Geometry check sheet. Reference: the model listing, model coordinates, mm. Face numbers are marked on the shaded views. Coordinates: 2 decimals unless noted, no trailing zeros. Write each loop counter-clockwise with the first axis right and the second up, starting at its lowest first coordinate (ties: lowest second). Pieces come first, ordered by that corner, then holes. Notation, with made-up numbers: (74.5, 40.5) -> (110.5, 40.5) arc R12 ccw to (110.5, 58.5) -> close; hole circle Ø5 at (12, -12). An arc over 180 degrees is marked (long way). Answer in a Markdown table with one row per item. Add a question column.
Q1. Thickness scan on line 1 (Y direction, x = 0, z = 1); line 2 (X direction, y = 1, z = 8.5); line 3 (Y direction, x = 0, z = 18). Record the ranges inside material, lowest first.
Q2. Gauge pin test, flat ends, axial feed: P1, Ø1, axis at x = 16, z = 15.5, coming from the +Y side; P2, Ø18, axis at x = 0, y = 158, coming from the +Z side (1 decimal); P3, Ø1, axis at x = 80, y = 16, coming from the -Z side; P4, Ø2, axis at x = 62.5, z = -7.5, coming from the -Y side. Record the tip position at first contact, or that the pin passes through.
Q3. Section check A-A, the plane x = 0. Record the boundary of the cut face in (y, z), and give its area (3 significant figures).
Q4. Section check B-B, the plane z = 15. Record the boundary of the cut face in (x, y), and give its area (3 significant figures).
Q5. Release check for a two-part mould opening along Y. For the marked faces 1, 2, 3 and 4 record: pulls with the +Y half, pulls with the -Y half, needs draft (parallel to the pull), parting line crosses it, or undercut.
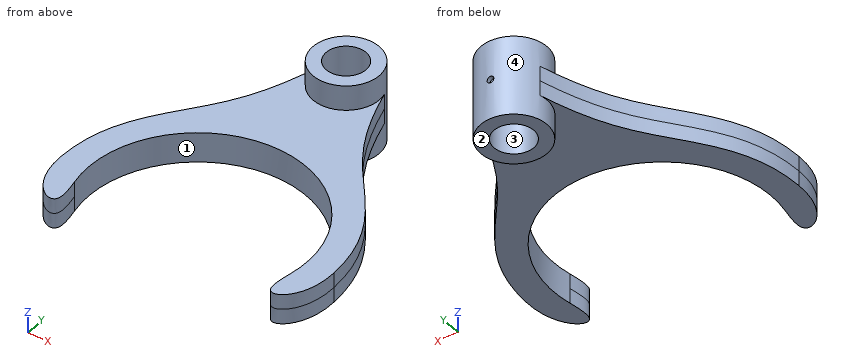
```python
from build123d import *

# Parameters (mm, degrees)
BOSS_EXTRUDE1_DEPTH = 11.25
SKETCH1_3_R         = 25
SKETCH1_3_R_2       = 15
BOSS_EXTRUDE2_DEPTH = 30
SKETCH3_R           = 2.5
CUT_EXTRUDE1_DEPTH  = 4


with BuildPart() as part:
    # Sketch1 → Boss-Extrude1 (new body, symmetric)
    with BuildSketch(Plane.XY):
        with BuildLine():
            ThreePointArc((-80.369346148, -16.271699348), (0, 82), (80.369346148, -16.271699348))
            add(Edge.make_bspline(
                [(101.737711244, 0), (102.498129601, -29.89988011), (76.506237686, -48.322432058), (78.198626966, -26.993338043), (80.369346148, -16.271699348)],
                knots=[0, 0, 0, 0, 0.676560131, 1, 1, 1, 1], degree=3))
            add(Edge.make_bspline(
                [(101.737711244, 0), (100.620263928, 43.938366918), (64.346417004, 80.312533322), (34.633446861, 126.224897928), (24.110391918, 164.609765621)],
                knots=[0, 0, 0, 0, 0.598565743, 1, 1, 1, 1], degree=3))
            ThreePointArc((24.110391918, 164.609765621), (24.776599827, 161.334681548), (25, 158))
            ThreePointArc((25, 158), (-3.334681548, 133.223400173), (-24.110391918, 164.609765621))
            add(Edge.make_bspline(
                [(-101.737711244, 0), (-100.620263928, 43.938366918), (-64.346417004, 80.312533322), (-34.633446861, 126.224897928), (-24.110391918, 164.609765621)],
                knots=[0, 0, 0, 0, 0.598565743, 1, 1, 1, 1], degree=3))
            add(Edge.make_bspline(
                [(-101.737711244, 0), (-102.498129601, -29.89988011), (-76.506237686, -48.322432058), (-78.198626966, -26.993338043), (-80.369346148, -16.271699348)],
                knots=[0, 0, 0, 0, 0.676560131, 1, 1, 1, 1], degree=3))
        make_face()
    extrude(amount=BOSS_EXTRUDE1_DEPTH, both=True)

    # Sketch1<3> → Boss-Extrude2 (add, symmetric)
    with BuildSketch(Plane.XY):
        with Locations((0, 158)):
            Circle(SKETCH1_3_R)
        with Locations((0, 158)):
            Circle(SKETCH1_3_R_2, mode=Mode.SUBTRACT)
    extrude(amount=BOSS_EXTRUDE2_DEPTH, both=True)

    # Sketch3 → Cut-Extrude1 (cut, through all)
    with BuildSketch(Plane(origin=(0, 180, 0), x_dir=(1, 0, 0), z_dir=(0, 1, 0))):
        Circle(SKETCH3_R)
    extrude(amount=CUT_EXTRUDE1_DEPTH, mode=Mode.SUBTRACT)


solid = part.part
```
Calculated:
| question | item | result |
|---|---|---|
| 1 | line 1 | y = 82 to 143, 173 to 180 |
| 1 | line 2 | x = -101.71 to -81.99, 81.99 to 101.71 |
| 1 | line 3 | y = 133 to 143, 173 to 183 |
| 2 | P1 | stops at y = 177.62 |
| 2 | P2 | passes through |
| 2 | P3 | stops at z = -11.25 |
| 2 | P4 | stops at y = 51.88 |
| 3 | outline | (82, -11.25) -> (133, -11.25) -> (133, -30) -> (143, -30) -> (143, 30) -> (133, 30) -> (133, 11.25) -> (82, 11.25) -> close; (173, -30) -> (183, -30) -> (183, -2.5) -> (180, -2.5) -> (180, 2.5) -> (183, 2.5) -> (183, 30) -> (173, 30) -> close |
| 3 | area | 2,330 mm² |
| 4 | outline | circle Ø50 at (0, 158); hole circle Ø30 at (0, 158) |
| 4 | area | 1,260 mm² |
| 5 | face 1 | undercut |
| 5 | face 2 | needs draft |
| 5 | face 3 | undercut |
| 5 | face 4 | parting line crosses it |
